Verification items for the finished model (mm, model axes). Face numbers are marked on the shaded views. A direction names the side the tool comes from. Round coordinates to 2 decimals unless told otherwise and drop trailing zeros. Order: outer loops, then holes, each group sorted by start corner. A loop starts at its lowest first (then second) coordinate and runs counter-clockwise, first axis right, second up. Notation, with made-up numbers: (11, -19) -> (22, -19) arc R9 cw to (22, -3) -> close; hole circle Ø3 at (25, -2). An arc over 180 degrees is marked (long way). Return JSON: item names as keys, results as strings. Group by question number.
Item 1: Sectioned sample at C-C on z = 8.25. Record the cut outline in (x, y).
Item 2: Scan lines: probe 1 along Z at (x, y) = (-3.25, -1); probe 2 along X at (y, z) = (2.5, 0.5); probe 3 along Y at (x, z) = (0, 7.25). Record each from-to range of solid material in increasing order. Write a range as from..to.
Item 3: Sectioned sample at D-D on y = 3.5. Record the cut outline in (x, z).
Item 4: Depth check by flat-ended pin: pin 1 Ø3 at (x, y) = (-4, -2.5) entering from +Z; pin 2 Ø1 at (y, z) = (-2, 4.5) entering from +X; pin 3 Ø1 at (x, z) = (-4, 2.5) entering from +Y; pin 4 Ø2 at (x, y) = (3.5, -2) entering from -Z. Enter the tip coordinate at first touch or a pass-through.
Item 5: Access from +Z, -Z, +X, -X, +Y, -Y to the whole of each face (thin tool, end or side, straight path). Record for the marked faces 1, 2 and 3.
Item 6: Sectioned sample at B-B on y = 0. Record the cut outline in (x, z), plus the area to 3 significant figures.
Item 7: Sectioned sample at A-A on x = 0. Record the cut outline in (y, z).
```python
from build123d import *

# Parameters (mm, degrees)
F0_R     = 1.75
F1_DEPTH = 0.4
F2_R     = 0.85
F3_DEPTH = 2.6
F5_DEPTH = 0.3
F6_SIZE2 = 0.3
F6_SIZE  = 0.3
F7_SCALE = 3


with BuildPart() as f1:
    # F0 (on Top) → F1 (new body)
    with BuildSketch(Plane.XY):
        Circle(F0_R)
    extrude(amount=F1_DEPTH)

    # F2 (on face) → F3 (join)
    with BuildSketch(Plane.XY.offset(0.4)):
        Circle(F2_R)
    extrude(amount=F3_DEPTH)

    # F4 (on face) → F5 (cut)
    with BuildSketch(Plane(origin=(0, 0, 0), x_dir=(1, 0, 0), z_dir=(0, 0, -1))):
        with BuildLine():
            ThreePointArc((0.25, 1.7320508076), (0, 1.75), (-0.25, 1.7320508076))
            Line((-0.25, 1.7320508076), (-0.25, -1.7320508076))
            ThreePointArc((-0.25, -1.7320508076), (0, -1.75), (0.25, -1.7320508076))
            Line((0.25, -1.7320508076), (0.25, 1.7320508076))
        make_face()
    extrude(amount=-F5_DEPTH, mode=Mode.SUBTRACT)

    # F6
    f6_edges = [f1.edges().sort_by_distance(p)[0] for p in [
        (-0.85, 0, 3),
    ]]
    chamfer(f6_edges, length=F6_SIZE, length2=F6_SIZE2)


with BuildPart() as f1_1:
    # F7: moved
    add(f1.part.scale(F7_SCALE))


solid = f1_1.part
```
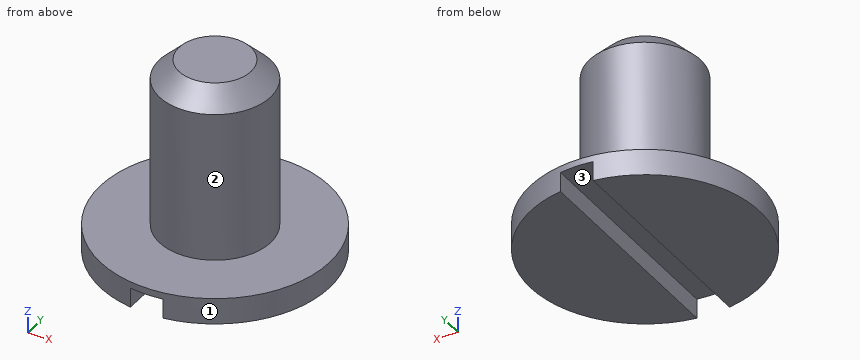
Recorded:
{
 "1": {"outline": "circle Ø4.8 at (0, 0)"},
 "2": {"probe 1": "0..1.2", "probe 2": "-4.62..-0.75, 0.75..4.62", "probe 3": "-2.55..2.55"},
 "3": {"outline": "(-3.91, 0) -> (-0.75, 0) -> (-0.75, 0.9) -> (0.75, 0.9) -> (0.75, 0) -> (3.91, 0) -> (3.91, 1.2) -> (-3.91, 1.2) -> close"},
 "4": {"pin 1": "z = 1.2", "pin 2": "x = 2.06", "pin 3": "through", "pin 4": "z = 0"},
 "5": {"face 1": "+Z, -Z", "face 2": "+Z", "face 3": "-Z, +Y, -Y"},
 "6": {"outline": "(-5.25, 0) -> (-0.75, 0) -> (-0.75, 0.9) -> (0.75, 0.9) -> (0.75, 0) -> (5.25, 0) -> (5.25, 1.2) -> (2.55, 1.2) -> (2.55, 8.1) -> (1.65, 9) -> (-1.65, 9) -> (-2.55, 8.1) -> (-2.55, 1.2) -> (-5.25, 1.2) -> close", "area": "50.2 mm²"},
 "7": {"outline": "(-5.25, 0.9) -> (5.25, 0.9) -> (5.25, 1.2) -> (2.55, 1.2) -> (2.55, 8.1) -> (1.65, 9) -> (-1.65, 9) -> (-2.55, 8.1) -> (-2.55, 1.2) -> (-5.25, 1.2) -> close"}
}
